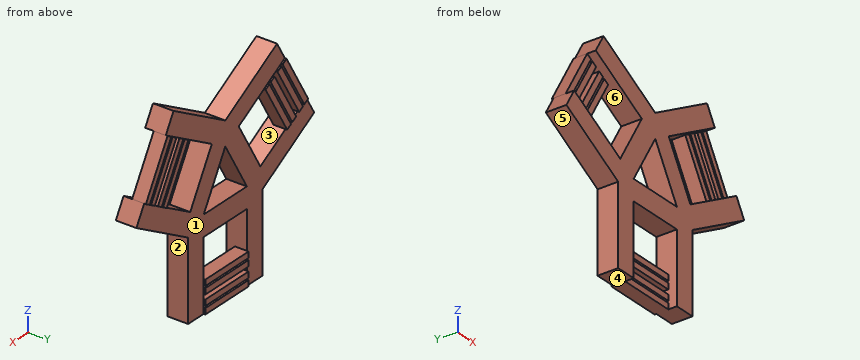
```python
from build123d import *

# Parameters (mm, degrees)
SALIENTE_EXTRUIR1_DEPTH   = 15
SALIENTE_EXTRUIR1_2_DEPTH = 15
SALIENTE_EXTRUIR1_3_DEPTH = 15
SALIENTE_EXTRUIR1_4_DEPTH = 15
SALIENTE_EXTRUIR1_5_DEPTH = 15
SALIENTE_EXTRUIR1_6_DEPTH = 15
CROQUIS1_4_W              = 125
CROQUIS1_4_H              = 25.75
CROQUIS1_4_W_2            = 250
SALIENTE_EXTRUIR2_DEPTH   = 30
SALIENTE_EXTRUIR3_DEPTH   = 22.5
SALIENTE_EXTRUIR4_DEPTH   = 67.5


with BuildPart() as part:
    # Croquis1 → Saliente-Extruir1 (new body, symmetric)
    with BuildSketch(Plane(origin=(0, 0, 0), x_dir=(1, 0, 0), z_dir=(0, 1, 0))):
        Polygon((-377.949753328, -73.871824527), (-315.449753328, -182.125), (-252.949753328, -290.378175473), (-245.588537396, -286.128175473), (-370.588537396, -69.621824527), align=None)
    extrude(amount=SALIENTE_EXTRUIR1_DEPTH, both=True)



with BuildPart() as body_2:
    # Croquis1 → Saliente-Extruir1 2 (new body, symmetric)
    with BuildSketch(Plane(origin=(0, 0, 0), x_dir=(1, 0, 0), z_dir=(0, 1, 0))):
        Polygon((-314.870569699, -326.128175473), (-377.370569699, -217.875), (-439.870569699, -109.621824527), (-447.231785631, -113.871824527), (-322.231785631, -330.378175473), align=None)
    extrude(amount=SALIENTE_EXTRUIR1_2_DEPTH, both=True)


with BuildPart() as body_3:
    # Croquis1 → Saliente-Extruir1 3 (new body, symmetric)
    with BuildSketch(Plane(origin=(0, 0, 0), x_dir=(1, 0, 0), z_dir=(0, 1, 0))):
        Polygon((-125, 364.25), (-125, 355.75), (125, 355.75), (125, 364.25), (0, 364.25), align=None)
    extrude(amount=SALIENTE_EXTRUIR1_3_DEPTH, both=True)


with BuildPart() as body_4:
    # Croquis1 → Saliente-Extruir1 4 (new body, symmetric)
    with BuildSketch(Plane(origin=(0, 0, 0), x_dir=(1, 0, 0), z_dir=(0, 1, 0))):
        Polygon((370.588537396, -69.621824527), (245.588537396, -286.128175473), (252.949753328, -290.378175473), (315.449753328, -182.125), (377.949753328, -73.871824527), align=None)
    extrude(amount=SALIENTE_EXTRUIR1_4_DEPTH, both=True)


with BuildPart() as body_5:
    # Croquis1 → Saliente-Extruir1 5 (new body, symmetric)
    with BuildSketch(Plane(origin=(0, 0, 0), x_dir=(1, 0, 0), z_dir=(0, 1, 0))):
        Polygon((-125, 444.25), (-125, 435.75), (0, 435.75), (125, 435.75), (125, 444.25), align=None)
    extrude(amount=SALIENTE_EXTRUIR1_5_DEPTH, both=True)


with BuildPart() as body_6:
    # Croquis1 → Saliente-Extruir1 6 (new body, symmetric)
    with BuildSketch(Plane(origin=(0, 0, 0), x_dir=(1, 0, 0), z_dir=(0, 1, 0))):
        Polygon((377.370569699, -217.875), (314.870569699, -326.128175473), (322.231785631, -330.378175473), (447.231785631, -113.871824527), (439.870569699, -109.621824527), align=None)
    extrude(amount=SALIENTE_EXTRUIR1_6_DEPTH, both=True)


with BuildPart() as part_1:
    add(part.part)

    add(body_2.part)  # Saliente-Extruir2 merges body 2

    add(body_3.part)  # Saliente-Extruir2 merges body 3

    add(body_4.part)  # Saliente-Extruir2 merges body 4

    add(body_5.part)  # Saliente-Extruir2 merges body 5

    add(body_6.part)  # Saliente-Extruir2 merges body 6
    # Croquis1_4 → Saliente-Extruir2 (add, symmetric)
    with BuildSketch(Plane(origin=(0, 0, 0), x_dir=(1, 0, 0), z_dir=(0, 1, 0))):
        with Locations((62.5, 422.875)):
            Rectangle(CROQUIS1_4_W, CROQUIS1_4_H)
        with Locations((0, 457.125)):
            Rectangle(CROQUIS1_4_W_2, CROQUIS1_4_H)
        with Locations((-62.5, 422.875)):
            Rectangle(CROQUIS1_4_W, CROQUIS1_4_H)
        with Locations((-62.5, 377.125)):
            Rectangle(CROQUIS1_4_W, CROQUIS1_4_H)
        with Locations((62.5, 377.125)):
            Rectangle(CROQUIS1_4_W, CROQUIS1_4_H)
        with Locations((0, 342.875)):
            Rectangle(CROQUIS1_4_W_2, CROQUIS1_4_H)
        Polygon((-322.231785631, -330.378175473), (-447.231785631, -113.871824527), (-469.531939779, -126.746824527), (-344.531939779, -343.253175473), align=None)
        Polygon((-292.570415552, -313.253175473), (-355.070415552, -205), (-377.370569699, -217.875), (-314.870569699, -326.128175473), align=None)
        Polygon((-377.370569699, -217.875), (-355.070415552, -205), (-417.570415552, -96.746824527), (-439.870569699, -109.621824527), align=None)
        Polygon((-337.749907476, -195), (-315.449753328, -182.125), (-377.949753328, -73.871824527), (-400.249907476, -86.746824527), align=None)
        Polygon((-348.288383249, -56.746824527), (-370.588537396, -69.621824527), (-245.588537396, -286.128175473), (-223.288383249, -273.253175473), align=None)
        Polygon((-252.949753328, -290.378175473), (-315.449753328, -182.125), (-337.749907476, -195), (-275.249907476, -303.253175473), align=None)
        Polygon((348.288383249, -56.746824527), (223.288383249, -273.253175473), (245.588537396, -286.128175473), (370.588537396, -69.621824527), align=None)
        Polygon((315.449753328, -182.125), (252.949753328, -290.378175473), (275.249907476, -303.253175473), (337.749907476, -195), align=None)
        Polygon((400.249907476, -86.746824527), (377.949753328, -73.871824527), (315.449753328, -182.125), (337.749907476, -195), align=None)
        Polygon((439.870569699, -109.621824527), (417.570415552, -96.746824527), (355.070415552, -205), (377.370569699, -217.875), align=None)
        Polygon((355.070415552, -205), (292.570415552, -313.253175473), (314.870569699, -326.128175473), (377.370569699, -217.875), align=None)
        Polygon((322.231785631, -330.378175473), (344.531939779, -343.253175473), (469.531939779, -126.746824527), (447.231785631, -113.871824527), align=None)
    extrude(amount=SALIENTE_EXTRUIR2_DEPTH, both=True)

    # Croquis1_5 → Saliente-Extruir3 (add)
    with BuildSketch(Plane(origin=(0, 0, 0), x_dir=(1, 0, 0), z_dir=(0, 1, 0))):
        Polygon((77.942286341, -189.337567297), (202.942286341, 27.168783649), (469.531939779, -126.746824527), (514.531939779, -48.804538186), (215, 124.130307876), (215, 470), (125, 470), (125, 162.168783649), (-125, 162.168783649), (-125, 470), (-215, 470), (-215, 124.130307876), (-514.531939779, -48.804538186), (-469.531939779, -126.746824527), (-202.942286341, 27.168783649), (-77.942286341, -189.337567297), (-344.531939779, -343.253175473), (-299.531939779, -421.195461814), (0, -248.260615752), (299.531939779, -421.195461814), (344.531939779, -343.253175473), align=None)
        Polygon((-125, 72.168783649), (125, 72.168783649), (0, -144.337567297), align=None, mode=Mode.SUBTRACT)
    extrude(amount=SALIENTE_EXTRUIR3_DEPTH)

    # Croquis1_6 → Saliente-Extruir4 (add)
    with BuildSketch(Plane(origin=(0, 0, 0), x_dir=(1, 0, 0), z_dir=(0, 1, 0))):
        Polygon((77.942286341, -189.337567297), (202.942286341, 27.168783649), (469.531939779, -126.746824527), (514.531939779, -48.804538186), (215, 124.130307876), (215, 470), (125, 470), (125, 162.168783649), (-125, 162.168783649), (-125, 470), (-215, 470), (-215, 124.130307876), (-514.531939779, -48.804538186), (-469.531939779, -126.746824527), (-202.942286341, 27.168783649), (-77.942286341, -189.337567297), (-344.531939779, -343.253175473), (-299.531939779, -421.195461814), (0, -248.260615752), (299.531939779, -421.195461814), (344.531939779, -343.253175473), align=None)
        Polygon((-125, 72.168783649), (125, 72.168783649), (0, -144.337567297), align=None, mode=Mode.SUBTRACT)
    extrude(amount=-SALIENTE_EXTRUIR4_DEPTH)


solid = part_1.part
```
Can you work these out from the model? Positions are in its coordinate system, mm. Face numbers are marked on the shaded views. A direction names the side the tool comes from. Round coordinates to 2 decimals unless told otherwise and drop trailing zeros. Loops run counter-clockwise (first coordinate to the right, second up) from the corner with the lowest first, then second, coordinate; pieces in that order, holes last.
Item 1: Suppose I cut it at A-A, the plane z = -176. Write out the boundary of the cut face in (x, y), then the cut area to 3 significant figures.
Item 2: Which directions (+Z, -Z, +X, -X, +Y, -Y) give clear straight access to the entire face, cutting with the end or side of a thin tool? Please do the marked faces 1, 2 and 3.
Item 3: If we mould it in two halves opening along X, with no side actions, what happens to the marked faces 4, 5 and 6? For each: +X half, -X half, draft (parallel to the pull), parting line (faces both ways), or undercut.
Item 4: Please list where these lines run through material, in increasing order: L1, parallel to Z at x = -123.5, y = 25.5; L2, parallel to X at y = -56.5, z = -297.5; L3, parallel to X at y = -26.5, z = 72.5.
Item 5: Suppose I cut it at C-C, the plane x = 37.5. State how many separate pieces and enclosed holes the cut face has, then the cut area to 3 significant figures.
Item 6: Suppose I cut it at D-D, the plane x = -264. Write out the boundary of the cut face in (y, z), then the cut area to 3 significant figures.
Item 7: Suppose I cut it at B-B, the plane y = -42.5. Write out the boundary of the cut face in (x, z).
Item 8: Will these pins go through, and if not, where does the flat tip stop? pin 1 Ø8 at (y, z) = (25.5, -375) entering from +X; pin 2 Ø4 at (y, z) = (-30.5, 108) entering from +X; pin 3 Ø4 at (x, z) = (61, 182.5) entering from +Y.
Reported:
1. outline: (-215, -67.5) - (-125, -67.5) - (-125, 22.5) - (-215, 22.5) - close; (125, -67.5) - (215, -67.5) - (215, 22.5) - (125, 22.5) - close
1. area: 16,200 mm2
2. face 1: +Y
2. face 2: -Z, +X, +Y, -Y
2. face 3: -Y
3. face 4: draft
3. face 5: -X half
3. face 6: undercut
4. L1: z = -470 to -444.25, -435.75 to -410, -390 to -364.25, -355.75 to -330
4. L2: x = -215 to -125, 125 to 215
4. L3: x = -500.85 to -375.57, -368.93 to -339.19, -145.4 to -41.48, 41.48 to 145.4, 339.19 to 368.93, 375.57 to 500.85
5. separate pieces: 4
5. enclosed holes: 0
5. area: 31,900 mm2
6. outline: (-67.5, -95.84) - (22.5, -95.84) - (22.5, 8.08) - (-67.5, 8.08) - close; (-67.5, 296.76) - (-30, 296.76) - (-30, 271.24) - (-15, 271.24) - (-15, 254.24) - (-30, 254.24) - (-30, 202.74) - (30, 202.74) - (30, 254.24) - (15, 254.24) - (15, 271.24) - (30, 271.24) - (30, 296.76) - (22.5, 296.76) - (22.5, 400.68) - (-67.5, 400.68) - close
6. area: 23,800 mm2
7. outline: (-514.53, 48.8) - (-215, -124.13) - (-215, -470) - (-125, -470) - (-125, -162.17) - (125, -162.17) - (125, -470) - (215, -470) - (215, -124.13) - (514.53, 48.8) - (469.53, 126.75) - (202.94, -27.17) - (77.94, 189.34) - (344.53, 343.25) - (299.53, 421.2) - (0, 248.26) - (-299.53, 421.2) - (-344.53, 343.25) - (-77.94, 189.34) - (-202.94, -27.17) - (-469.53, 126.75) - close; hole (-125, -72.17) - (125, -72.17) - (0, 144.34) - close
8. pin 1: stops at x = 215
8. pin 2: stops at x = 481.51
8. pin 3: stops at y = 22.5
